Input: part model. Units: mm. Frame: model coordinates. Coordinates: 2 decimals unless noted, no trailing zeros. Write each loop counter-clockwise with the first axis right and the second up, starting at its lowest first coordinate (ties: lowest second). Pieces come first, ordered by that corner, then holes. Notation, with made-up numbers: (-10.5, -33) - (14.5, -33) arc R6 cw to (14.5, -27) - close; hole circle Ø10 at (65.5, 45.5). An arc over 180 degrees is marked (long way). Use a Markdown table: item, result. Add a question column.
Q1. Pin query (flat end, axial travel): P1, Ø1, axis at y = -108.5, z = 2, coming from the +X side; P2, Ø1, axis at y = -64.5, z = 1.5, coming from the +X side; P3, Ø1.6, axis at y = -67, z = 2.5, coming from the -X side. Return the tip coordinate at first contact, or that it passes through.
Q2. Section query D-D (y = -60). Return the cut outline in (x, z) (3 decimals).
Q3. Section query A-A (x = 30). Return the cut outline in (y, z) (3 decimals), then the cut area to 3 significant figures.
Q4. Section query B-B (y = -110.5). Return the cut outline in (x, z) (3 decimals), then the cut area to 3 significant figures.
Q5. Material intervals for probe 1 along X at (y, z) = (-118, 2.55) (3 decimals); probe 2 along Y at (x, z) = (18.5, 1.8); probe 3 along X at (y, z) = (-61, 2.8), sorted ascending. Write a range as from..to.
Q6. Section query C-C (z = 1.45). Return the cut outline in (x, y) (3 decimals).
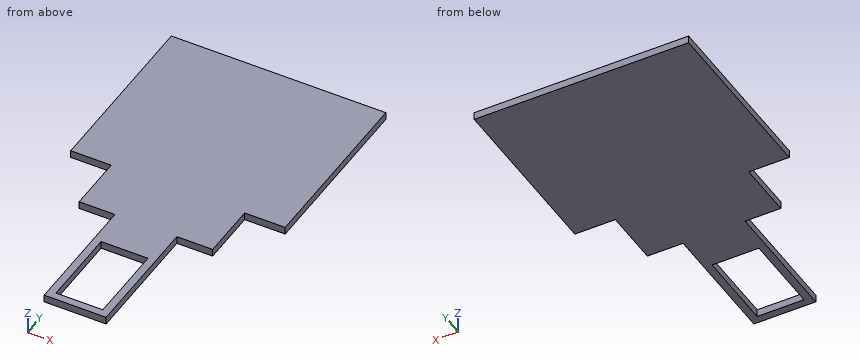
from build123d import *

# Parameters (mm, degrees)
F0_W     = 3.175
F0_H     = 25.4
F0_H_2   = 33.8328
F0_H_3   = 3.175
F1_DEPTH = 3.175
F2_DEPTH = 25.4


# Not quite as in the source:
# - a length typed as a fraction of an inch, garbled in the dataset ("3 / 203.2 mm" for 3/8 in), is restored


with BuildPart() as f1:
    # F0 (on Top) → F1 (new body)
    with BuildSketch(Plane.XY):
        Polygon((-13.825, 0), (0, 0), (56, 0), (69.825, 0), (69.825, 25.4), (-13.825, 25.4), align=None)
        Polygon((56, 0), (0, 0), (0, -23), (0, -50), (0, -74), (15, -74), (28, -74), (41, -74), (56, -74), (56, -50), (56, -23), align=None)
        Polygon((0, -23), (0, 0), (-13.825, 0), (-17, 0), (-17, -50), (0, -50), align=None)
        Polygon((69.825, 0), (56, 0), (56, -23), (56, -50), (73, -50), (73, 0), align=None)
        with Locations((-15.4125, 12.7)):
            Rectangle(F0_W, F0_H)
        with Locations((71.4125, 12.7)):
            Rectangle(F0_W, F0_H)
        Polygon((28, -74), (15, -74), (15, -90), (18.175, -90), (21.35, -90), (28, -90), (34.65, -90), (37.825, -90), (41, -90), (41, -74), align=None)
        with Locations((16.5875, -106.9164)):
            Rectangle(F0_W, F0_H_2)
        with Locations((39.4125, -106.9164)):
            Rectangle(F0_W, F0_H_2)
        with Locations((16.5875, -125.4203)):
            Rectangle(F0_W, F0_H_3)
        with Locations((39.4125, -125.4203)):
            Rectangle(F0_W, F0_H_3)
        Polygon((21.35, -123.8328), (18.175, -123.8328), (18.175, -127.0078), (37.825, -127.0078), (37.825, -123.8328), (34.65, -123.8328), align=None)
    extrude(amount=F1_DEPTH)

    # F0 (on Top) → F2 (cut)
    with BuildSketch(Plane.XY):
        Polygon((28, -90), (21.35, -90), (21.35, -123.8328), (34.65, -123.8328), (34.65, -90), align=None)
    extrude(amount=-F2_DEPTH, mode=Mode.SUBTRACT)


solid = f1.part
Values follow:
| question | item | result |
|---|---|---|
| 1 | P1 | x = 41 |
| 1 | P2 | x = 56 |
| 1 | P3 | x = 0 |
| 2 | outline | (0, 0) - (56, 0) - (56, 3.175) - (0, 3.175) - close |
| 3 | outline | (-127.008, 0) - (-123.833, 0) - (-123.833, 3.175) - (-127.008, 3.175) - close; (-90, 0) - (25.4, 0) - (25.4, 3.175) - (-90, 3.175) - close |
| 3 | area | 376 mm2 |
| 4 | outline | (15, 0) - (18.175, 0) - (18.175, 3.175) - (15, 3.175) - close; (37.825, 0) - (41, 0) - (41, 3.175) - (37.825, 3.175) - close |
| 4 | area | 20.2 mm2 |
| 5 | probe 1 | 15..18.175, 37.825..41 |
| 5 | probe 2 | -127.01..-123.83, -90..25.4 |
| 5 | probe 3 | 0..56 |
| 6 | outline | (-17, -50) - (0, -50) - (0, -74) - (15, -74) - (15, -127.008) - (41, -127.008) - (41, -74) - (56, -74) - (56, -50) - (73, -50) - (73, 25.4) - (-17, 25.4) - close; hole (18.175, -123.833) - (37.825, -123.833) - (37.825, -90) - (18.175, -90) - close |
